The listing builds one solid part. Answer for the finished solid, in the listing's coordinates (mm). A direction names the side the tool comes from. Give positions to 0.01 mm unless a question says otherwise; leave off trailing zeros. Write each loop counter-clockwise with the first axis right and the second up, starting at its lowest first coordinate (ties: lowest second). Pieces come first, ordered by that corner, then holes. Notation, with made-up numbers: (30, 56) -> (86, 56) arc R26 cw to (86, 83) -> close; hole circle Ø3 at (-20, 84). An arc over 180 degrees is marked (long way). Put each result on its own line as item: value. Start each with the question number.
1) For a pull along X with two mould halves and no side action, classify faces 1 (the flat face through (0, 0, 0)), 2 (the flat face through (0.51, -0.86, 17.26)), 3 (the cylindrical face through (-1.5, -0.07, 8.01)), 4 (the flat face through (-0.51, 0.86, 17.26)) as released by +X, released by -X, zero draft, split by the parting line, or undercut.
2) For faces 5 (the flat face through (0, 0, 16.5)), 6 (the flat face through (1.3, 0, 18)), determine the directions among +Z, -Z, +X, -X, +Y, -Y from which every point of the face is accessible in a straight line to the end or side of a thin tool.
3) Flat-ended cylindrical pins translate along their axes: pin 1 Ø0.6 at (y, z) = (0.5, 17.5) entering from +X; pin 2 Ø2 at (y, z) = (-2, 11) entering from +X; pin 3 Ø1.6 at (x, y) = (0.5, 0.5) entering from +Z; pin 4 Ø3 at (y, z) = (-1.5, 10.5) entering from -X. Find the tip coordinate at first contact, or state that the pin passes through.
4) A cutting plane is placed at B-B (z = 14.25). Write down the section's boundary in (x, y), then the cut area to 3 significant figures.
5) Find the intervals of material crossed by line 1 along Z through (x, y) = (-0.3, 0.55); line 2 along X through (y, z) = (0, 6), in increasing order. Write a range as from..to.
Autodesk Inventor part; units mm, degrees
ref_plane "YZ Plane" through (0, 0, 0) normal (1, 0, 0) x (0, 1, 0)
ref_plane "XZ Plane" through (0, 0, 0) normal (0, 1, 0) x (-1, 0, 0)
ref_plane "XY Plane" through (0, 0, 0) normal (0, 0, 1) x (1, 0, 0)
sketch "スケッチ1" plane through (0, 0, 0) normal (0, 0, 1) x (1, 0, 0)
  circle A0 centre (0, 0) radius 1.5
  dimension "d0" = 3
extrude "押し出し1" add sketch "スケッチ1" along normal blind 18
thread "ねじ1"
sketch "スケッチ2" plane through (0, 0, 18) normal (0, 0, 1) x (1, 0, 0)
  circle A0 centre (0, 0) radius 3
  dimension "d5" = 6
extrude "押し出し2" add sketch "スケッチ2" against normal blind 1.75
chamfer "面取り1" distance 1.5 angle 45 1 edges at (-3, 0, 16.25)
sketch "スケッチ3" plane through (0, 0, 18) normal (0, 0, 1) x (1, 0, 0)
  line L0 (0, 1.1547) -> (1, 0.5774)
  line L1 (1, 0.5774) -> (1, -0.5774)
  line L2 (1, -0.5774) -> (0, -1.1547)
  line L3 (0, -1.1547) -> (-1, -0.5774)
  line L4 (-1, -0.5774) -> (-1, 0.5774)
  line L5 (-1, 0.5774) -> (0, 1.1547)
  point P0 (0, 0)
  point P1 (0, 0)
  dimension "d11" = 2
extrude "押し出し3" cut sketch "スケッチ3" against normal blind 1.5
properties part number "m3皿ネジ18 (1)" material "鉄 灰色"
Reply:
1. face 1: zero draft
1. face 2: undercut
1. face 3: split by the parting line
1. face 4: undercut
2. face 5: +Z
2. face 6: +Z, +X, -X, +Y, -Y
3. pin 1: stops at x = 2.98
3. pin 2: stops at x = 1.12
3. pin 3: stops at z = 18
3. pin 4: stops at x = -1.5
4. outline: circle Ø3 at (0, 0)
4. area: 7.07 mm2
5. line 1: z = 0..16.5
5. line 2: x = -1.5..1.5
